from build123d import *

# Parameters (mm, degrees)
BOSS_EXTRUDE1_DEPTH = 10
SKETCH4_R           = 6
CUT_EXTRUDE1_DEPTH  = 2
SKETCH5_R           = 3.2
CUT_EXTRUDE2_DEPTH  = 131.441517879
CHAMFER1_SIZE       = 0.5


with BuildPart() as part:
    # Sketch3 → Boss-Extrude1 (new body)
    with BuildSketch(Plane.XY):
        with BuildLine():
            Line((-6.355283539, -23.287979746), (3.644716461, -83.287979746))
            ThreePointArc((3.644716461, -83.287979746), (10.445097015, -95.260399649), (23.372594937, -100))
            Line((23.372594937, -100), (53.372594937, -100))
            ThreePointArc((53.372594937, -100), (66.30009286, -95.260399649), (73.100473414, -83.287979746))
            Line((73.100473414, -83.287979746), (83.100473414, -23.287979746))
            ThreePointArc((83.100473414, -23.287979746), (78.632994587, -7.072502077), (63.372594937, 0))
            Line((63.372594937, 0), (13.372594937, 0))
            ThreePointArc((13.372594937, 0), (-1.887804712, -7.072502077), (-6.355283539, -23.287979746))
        make_face()
    extrude(amount=BOSS_EXTRUDE1_DEPTH)

    # Sketch4 → Cut-Extrude1 (cut)
    with BuildSketch(Plane.XY.offset(10)):
        with Locations((38.372594937, -25)):
            Circle(SKETCH4_R)
        with Locations((38.372594937, -75)):
            Circle(SKETCH4_R)
    extrude(amount=-CUT_EXTRUDE1_DEPTH, mode=Mode.SUBTRACT)

    # Sketch5 → Cut-Extrude2 (cut, through all)
    with BuildSketch(Plane.XY.offset(8)):
        with Locations((38.372594937, -25)):
            Circle(SKETCH5_R)
        with Locations((38.372594937, -75)):
            Circle(SKETCH5_R)
    extrude(amount=-CUT_EXTRUDE2_DEPTH, mode=Mode.SUBTRACT)

    # Chamfer1
    chamfer1_edges = [part.edges().sort_by_distance(p)[0] for p in [
        (66.30009286, -95.260399649, 0),
        (38.372594937, -100, 0),
        (10.445097015, -95.260399649, 0),
        (-1.355283539, -53.287979746, 0),
        (38.372594937, -100, 10),
        (66.30009286, -95.260399649, 10),
        (78.100473414, -53.287979746, 10),
        (78.632994587, -7.072502077, 10),
        (32.372594937, -25, 10),
        (32.372594937, -75, 10),
        (38.372594937, 0, 10),
        (-1.887804712, -7.072502077, 10),
        (35.172594937, -25, 0),
        (35.172594937, -75, 0),
        (-1.355283539, -53.287979746, 10),
        (-1.887804712, -7.072502077, 0),
        (10.445097015, -95.260399649, 10),
        (38.372594937, 0, 0),
        (78.632994587, -7.072502077, 0),
        (78.100473414, -53.287979746, 0),
    ]]
    chamfer(chamfer1_edges, length=CHAMFER1_SIZE)


solid = part.part
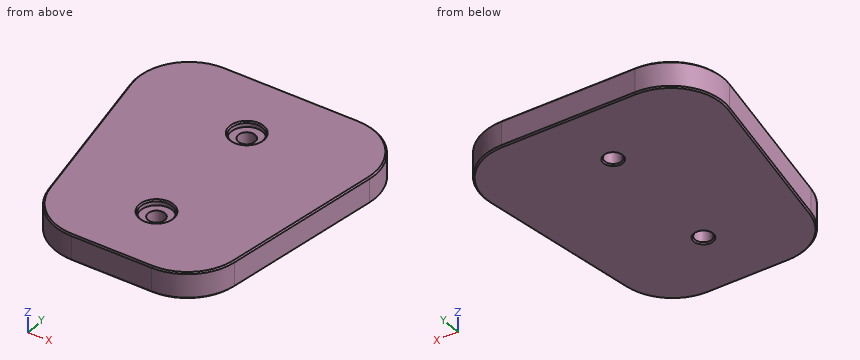
Source: CAD feature listing. Evaluate the final solid. Frame: model axes, mm. Give positions to 0.01 mm unless a question says otherwise; leave off trailing zeros. Order: outer loops, then holes, each group sorted by start corner. A loop starts at its lowest first (then second) coordinate and runs counter-clockwise, first axis right, second up. Notation, with made-up numbers: (80.5, 58.25) -> (93.5, 58.25) arc R9 cw to (93.5, 65.25) -> close; hole circle Ø3 at (8.25, -29.75). An arc over 180 degrees is marked (long way). Write item = value, one per line.
Item 1: Ray query, probe 1 along Y at (x, z) = (36.5, 5); probe 2 along X at (y, z) = (-23.5, 6.5); probe 3 along X at (y, z) = (-24.5, 9.75). Return the intervals inside material, ascending.
Check result:
probe_1 = -100 to -77.59, -72.41 to -27.59, -22.41 to 0
probe_2 = -6.32 to 35.55, 41.2 to 83.07
probe_3 = -5.9 to 32.14, 44.6 to 82.65
Item 2: Section query C-C (y = -25). Output: boundary loops of the cut face in (x, z).
Check result:
outline = (-6.07, 0.5) -> (-5.56, 0) -> (34.67, 0) -> (35.17, 0.5) -> (35.17, 8) -> (32.37, 8) -> (32.37, 9.5) -> (31.87, 10) -> (-5.56, 10) -> (-6.07, 9.5) -> close; (41.57, 0.5) -> (42.07, 0) -> (82.31, 0) -> (82.82, 0.5) -> (82.82, 9.5) -> (82.31, 10) -> (44.87, 10) -> (44.37, 9.5) -> (44.37, 8) -> (41.57, 8) -> close
Item 3: Contact query for flat-ended pins moving along their axis: pin 1 (4 mm diameter, centred on x = 65, z = 8.5, fed in from -Y); pin 2 (1 mm diameter, centred on y = -61, z = 2.5, fed in from -X); pin 3 (9.5 mm diameter, centred on x = 38.37, y = -25, fed in from +Z). Output: stop coordinate, or through.
Check result:
pin_1 = -97.53
pin_2 = -0.15
pin_3 = 8
Item 4: Section query A-A (z = 4.75). Output: boundary loops of the cut face in (x, y).
Check result:
outline = (-6.36, -23.29) -> (3.64, -83.29) arc R20 ccw to (23.37, -100) -> (53.37, -100) arc R20 ccw to (73.1, -83.29) -> (83.1, -23.29) arc R20 ccw to (63.37, 0) -> (13.37, 0) arc R20 ccw to start; hole circle Ø6.4 at (38.37, -75); hole circle Ø6.4 at (38.37, -25)
Item 5: Section query B-B (y = -75). Output: boundary loops of the cut face in (x, z), then the cut area to 3 significant figures.
Check result:
outline = (2.26, 0.5) -> (2.77, 0) -> (34.67, 0) -> (35.17, 0.5) -> (35.17, 8) -> (32.37, 8) -> (32.37, 9.5) -> (31.87, 10) -> (2.77, 10) -> (2.26, 9.5) -> close; (41.57, 0.5) -> (42.07, 0) -> (73.97, 0) -> (74.48, 0.5) -> (74.48, 9.5) -> (73.97, 10) -> (44.87, 10) -> (44.37, 9.5) -> (44.37, 8) -> (41.57, 8) -> close
area = 646 mm²
